Read the model definition and answer for the solid it produces. Units are mm, in the model's axes. A direction names the side the tool comes from. Coordinates: 2 decimals unless noted, no trailing zeros. Order: outer loops, then holes, each group sorted by start corner. A loop starts at its lowest first (then second) coordinate and runs counter-clockwise, first axis right, second up. Notation, with made-up numbers: (9, 50) -> (60, 50) arc R28 cw to (60, 88) -> close; hole circle Ø7 at (83, -3). An arc over 180 degrees is marked (long way). Return JSON: item names as keys, results as strings. Group by question number.
```python
from build123d import *

# Parameters (mm, degrees)
SKETCH_1_R      = 4.75
EXTRUDE_1_DEPTH = 19.5
EXTRUDE_2_DEPTH = 22.5


with BuildPart() as part:
    # 草图1 → 凸台-拉伸1 (new body)
    with BuildSketch(Plane(origin=(0, 0, 0), x_dir=(1, 0, 0), z_dir=(0, 1, 0))):
        with Locations(Location((0, 0, 0), (0, 0, 270))):
            Circle(SKETCH_1_R)
    extrude(amount=EXTRUDE_1_DEPTH)

    # 草图2 → 凸台-拉伸2 (add)
    with BuildSketch(Plane(origin=(0, 19.5, 0), x_dir=(1, 0, 0), z_dir=(0, 1, 0))):
        with BuildLine():
            ThreePointArc((2.5, 0), (-1.118033989, 2.236067977), (-1.5, -2))
            Line((-1.5, -2), (1.5, -2))
            ThreePointArc((1.5, -2), (2.236067977, -1.118033989), (2.5, 0))
        make_face()
    extrude(amount=EXTRUDE_2_DEPTH)


solid = part.part
```
1. Which of the six approach directions +Z, -Z, +X, -X, +Y, -Y give full straight-line access (tool end or side, diameter ignored) to faces 1 (the face through (0, 31, 2)), 2 (the face through (-2, 19.5, 2)), 3 (the face through (0, 0, 0))?
2. Find section D-D on y = 31. Determine the outline of the cut face in (x, z).
3. Find section A-A on x = 0. Determine the outline of the cut face in (y, z).
4. Find section C-C on z = 0.75. Determine the outline of the cut face in (x, y).
5. Given pin 1 (1.5 mm diameter, centred on x = -1, y = 14, fed in from -Z); pin 2 (4 mm diameter, centred on y = 21, z = -3, fed in from -X); pin 3 (3 mm diameter, centred on x = 2, y = 19, fed in from +Z), each flat-ended and moving along its own axis, determine where each tip first touches the part or whether it passes through.
6. Straight lines are drawn through the part: L1, parallel to Y at x = 2.5, z = -1.5; L2, parallel to Z at x = 2, y = 38.5; L3, parallel to Z at x = -2.5, y = 9. For each, find the intervals that lie inside material, in ascending order.
7. Find section B-B on y = 8. Determine the outline of the cut face in (x, z), and give its area (3 significant figures).
Result:
{
 "1": {"face 1": "+Z, +X, -X, +Y", "face 2": "+Y", "face 3": "+Z, -Z, +X, -X, -Y"},
 "2": {"outline": "(-1.5, 2) arc R2.5 ccw (long way) to (1.5, 2) -> close"},
 "3": {"outline": "(0, -4.75) -> (19.5, -4.75) -> (19.5, -2.5) -> (42, -2.5) -> (42, 2) -> (19.5, 2) -> (19.5, 4.75) -> (0, 4.75) -> close"},
 "4": {"outline": "(-4.69, 0) -> (4.69, 0) -> (4.69, 19.5) -> (2.38, 19.5) -> (2.38, 42) -> (-2.38, 42) -> (-2.38, 19.5) -> (-4.69, 19.5) -> close"},
 "5": {"pin 1": "z = -4.74", "pin 2": "x = -4.44", "pin 3": "z = 4.72"},
 "6": {"L1": "0 to 19.5", "L2": "-1.5 to 1.5", "L3": "-4.04 to 4.04"},
 "7": {"outline": "circle Ø9.5 at (0, 0)", "area": "70.9 mm^2"}
}
